from build123d import *

# Parameters (mm, degrees)
F1_DEPTH = 44.45
F3_DEPTH = 44.45
F5_START = -9.525
F5_DEPTH = 25.4
F6_R     = 19.04999
F7_SIZE2 = 12.69999
F7_SIZE  = 12.69999


# Not quite as in the source:
# - a fillet or chamfer is up to 0.001 mm smaller than in the source, because OpenCascade refuses the exact size


with BuildPart() as f1:
    # F0 (on Front) → F1 (new body)
    with BuildSketch(Plane.XZ):
        Polygon((-19.05, -44.0120689886), (0, -44.0120689886), (19.05, -44.0120689886), (19.05, 108.3879310114), (-19.05, 108.3879310114), align=None)
    extrude(amount=F1_DEPTH)

    # F2 (on face) → F3 (join)
    with BuildSketch(Plane.XZ.offset(44.45)):
        Polygon((-25.4, 108.3879310114), (-19.05, 108.3879310114), (19.05, 108.3879310114), (25.4, 108.3879310114), (25.4, 121.0879310114), (-25.4, 121.0879310114), align=None)
    extrude(amount=-F3_DEPTH)

    # F4 (on face) → F5 (join)
    with BuildSketch(Plane.XZ.offset(44.45).offset(F5_START)):
        with BuildLine():
            Line((-19.05, 273.4879310114), (-19.05, 121.0879310114))
            Line((-19.05, 121.0879310114), (19.05, 121.0879310114))
            Line((19.05, 121.0879310114), (19.05, 273.4879310114))
            ThreePointArc((19.05, 273.4879310114), (-37.5025933071, 530.403553002), (0, 790.7828688622))
            Line((0, 790.7828688622), (-19.05, 842.4347043037))
            ThreePointArc((-19.05, 842.4347043037), (-83.1207001827, 557.9613176576), (-19.05, 273.4879310114))
        make_face()
    extrude(amount=-F5_DEPTH)

    # F6 (radius 19.05 in the source; OpenCascade refuses exactly that, so slightly less here)
    f6_edges = [f1.edges().sort_by_distance(p)[0] for p in [
        (19.05, 0, 32.187931),
        (19.05, -44.45, 32.187931),
        (-19.05, -44.45, 32.187931),
        (-19.05, 0, 32.187931),
    ]]
    fillet(f6_edges, radius=F6_R)

    # F7 (size 12.7 and 12.7 in the source; OpenCascade refuses exactly that, so slightly less here)
    f7_edges = [f1.edges().sort_by_distance(p)[0] for p in [
        (-37.502593, -34.925, 530.403553),
        (-37.502593, -9.525, 530.403553),
        (-83.1207, -34.925, 557.961318),
        (-83.1207, -9.525, 557.961318),
        (-9.525, -34.925, 816.608787),
        (-9.525, -9.525, 816.608787),
        (-19.05, -34.925, 197.287931),
        (-19.05, -9.525, 197.287931),
        (19.05, -34.925, 197.287931),
        (19.05, -9.525, 197.287931),
    ]]
    chamfer(f7_edges, length=F7_SIZE, length2=F7_SIZE2)


solid = f1.part
Input: part model. Units: mm. Frame: model coordinates. A direction names the side the tool comes from. Give positions to 0.01 mm unless a question says otherwise; leave off trailing zeros. Use one line per item in the form item = value.
1. Reachability of faces 4 (the face through (-21, -23, 108.388)), 5 (the face through (13.32, -39.02, 33.25)), 6 (the face through (-13.62, -5.73, 31.12)), 7 (the face through (13.32, -5.43, 33.25)) from +Z, -Z, +X, -X, +Y, -Y: full face, straight path, thin tool, end or side. Return the list, or none.
Outcome:
face_4 = -Z, -X
face_5 = -Z, +X, -Y
face_6 = -Z, -X, +Y
face_7 = -Z, +X, +Y
2. First-contact query: P1, Ø4, axis at x = 0.5, z = 261, coming from the -Y side (3 decimals); P2, Ø8, axis at y = -31, z = 207.5, coming from the +X side (3 decimals); P3, Ø3, axis at y = -23.5, z = 36.5, coming from the -X side. Flat tips, straight axial feed; report the tip coordinate or a pass-through.
Outcome:
P1 = -34.925
P2 = 14.275
P3 = -19.05
3. Mould query, pull axis Z, two halves, no side actions, for faces 1 (the face through (0, -22, -44.012)), 2 (the face through (-38.15, -21.43, 526.67)), 3 (the face through (-13.32, -39.02, 31.12)). Classes: released by +Z, released by -Z, zero draft, split by the parting line, or undercut.
Outcome:
face_1 = released by -Z
face_2 = undercut
face_3 = zero draft
4. Ray query, L1, parallel to X at y = -22.5, z = 80; L2, parallel to Z at x = -13, y = -7.5; L3, parallel to Z at x = -16, y = -4. Return the intervals inside material, ascending.
Outcome:
L1 = -19.05 to 19.05
L2 = -44.01 to 121.09
L3 = 108.39 to 121.09
